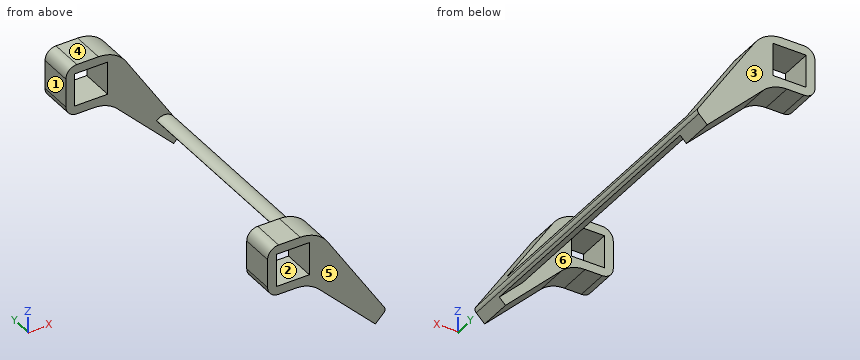
from build123d import *

# Parameters (mm, degrees)
SKETCH_1_W          = 15.000000000000002
SKETCH_1_H          = 15
EXTRUDE_1_DEPTH     = 160
CUT_EXTRUDE_2_DEPTH = 35
FILLET_3_R          = 5
FILLET_4_R          = 5
FILLET_6_R          = 15
FILLET_7_R          = 15
FILLET_8_R          = 15
FILLET_9_R          = 15
EXTRUDE_2_DEPTH     = 159
FILLET_10_R         = 5
FILLET_11_R         = 2


with BuildPart() as part:
    # Sketch 1 → Extrude 1 (new body)
    with BuildSketch(Plane(origin=(0, 0, 0), x_dir=(1, 0, 0), z_dir=(0, 1, 0))):
        Polygon((-11.5, 11.500000000000002), (7.5, 11.500000000000002), (37.49999999999999, 41.49999999999999), (42.44974746830583, 36.550252531694156), (11.5, -11.5), (-11.5, -11.5), align=None)
        Rectangle(SKETCH_1_W, SKETCH_1_H, mode=Mode.SUBTRACT)
    extrude(amount=EXTRUDE_1_DEPTH)

    # Sketch 4 → Cut-Extrude 2 (cut, symmetric)
    with BuildSketch(Plane(origin=(0, 0, -11.500000000000002), x_dir=(-1, 0, 0), z_dir=(0, 0, -1))):
        Polygon((-62.54884054332868, 145.00000000000003), (52.803582628705634, 145.00000000000003), (52.80358262870564, 15), (-62.548840543328666, 15), align=None)
    extrude(amount=CUT_EXTRUDE_2_DEPTH, both=True, mode=Mode.SUBTRACT)


with BuildPart() as cut_extrude_2_piece_1:
    # of the separate pieces the step leaves, piece 1, a body of its own (cut_extrude_2_pieces)
    add(part.part.solids().sort_by_distance((-11.5, 0, -11.5))[0])

    # Fillet 4
    fillet_4_edges = [cut_extrude_2_piece_1.edges().sort_by_distance(p)[0] for p in [
        (-11.5, 7.5, 11.5),
        (-11.5, 7.5, -11.500000000000002),
    ]]
    fillet(fillet_4_edges, radius=FILLET_4_R)

    # Fillet 7
    fillet_7_edges = [cut_extrude_2_piece_1.edges().sort_by_distance(p)[0] for p in [
        (11.5, 7.5, 11.5),
    ]]
    fillet(fillet_7_edges, radius=FILLET_7_R)

    # Fillet 8
    fillet_8_edges = [cut_extrude_2_piece_1.edges().sort_by_distance(p)[0] for p in [
        (7.5, 7.5, -11.500000000000002),
    ]]
    fillet(fillet_8_edges, radius=FILLET_8_R)



with BuildPart() as cut_extrude_2_piece_2:
    # of the separate pieces the step leaves, piece 2, a body of its own (cut_extrude_2_pieces)
    add(part.part.solids().sort_by_distance((7.5, 145, -11.5))[0])

    # Fillet 3
    fillet_3_edges = [cut_extrude_2_piece_2.edges().sort_by_distance(p)[0] for p in [
        (-11.5, 152.5, -11.500000000000002),
        (-11.5, 152.5, 11.5),
    ]]
    fillet(fillet_3_edges, radius=FILLET_3_R)

    # Fillet 6
    fillet_6_edges = [cut_extrude_2_piece_2.edges().sort_by_distance(p)[0] for p in [
        (11.5, 152.5, 11.5),
    ]]
    fillet(fillet_6_edges, radius=FILLET_6_R)

    # Fillet 9
    fillet_9_edges = [cut_extrude_2_piece_2.edges().sort_by_distance(p)[0] for p in [
        (7.5, 152.5, -11.500000000000002),
    ]]
    fillet(fillet_9_edges, radius=FILLET_9_R)


with BuildPart() as cut_extrude_2_piece_1_1:
    add(cut_extrude_2_piece_1.part)

    add(cut_extrude_2_piece_2.part)  # Extrude 2 merges Cut-Extrude 2 piece 2
    # Sketch 6 → Extrude 2 (add)
    with BuildSketch(Plane.XZ):
        Polygon((29.72182540693865, -28.064971157451247), (34.139072919876334, -23.647723644513547), (42.44974746830049, -36.550252531685864), (40.328427124736876, -38.671572875249474), align=None)
    extrude(amount=-EXTRUDE_2_DEPTH)

    # Fillet 10
    fillet_10_edges = [cut_extrude_2_piece_1_1.edges().sort_by_distance(p)[0] for p in [
        (34.139072919876334, 80.00000000000003, -23.647723644513547),
    ]]
    fillet(fillet_10_edges, radius=FILLET_10_R)

    # Fillet 11
    fillet_11_edges = [cut_extrude_2_piece_1_1.edges().sort_by_distance(p)[0] for p in [
        (42.449747468304494, 80, -36.55025253169208),
    ]]
    fillet(fillet_11_edges, radius=FILLET_11_R)


solid = cut_extrude_2_piece_1_1.part
The model under review builds one solid part; all positions refer to its coordinate system, in mm. Face numbers are marked on the shaded views. A direction names the side the tool comes from. Round coordinates to 2 decimals unless told otherwise and drop trailing zeros. Write each loop counter-clockwise with the first axis right and the second up, starting at its lowest first coordinate (ties: lowest second). Pieces come first, ordered by that corner, then holes. Notation, with made-up numbers: M -10,83.25 L 38,83.25 A25 ccw 38,103.25 Z; hole C -4,-39.75 d3. An arc over 180 degrees is marked long. Use a Markdown table: item, result. Add a question column.
Q1. To check wall thickness, follow line 1 (Y direction, x = 16.5, z = -14); line 2 (X direction, y = 12, z = -7); line 3 (X direction, y = 124.5, z = -34). State the ranges of each line that lie inside material, in increasing order.
Q2. We need section B-B, the plane z = -13. State the section outline as (x, y) points, plus the area to 3 significant figures.
Q3. Insertion check: pin 1 (6 mm diameter, centred on x = -1.5, y = 152, fed in from -Z); pin 2 (12 mm diameter, centred on x = -2.5, y = 4, fed in from -Z); pin 3 (16.5 mm diameter, centred on y = 11, z = 3, fed in from +X). Each pin has a flat end and moves straight along its axis. Give the tip position at first contact, or say it passes through.
Q4. We need section D-D, the plane z = -2. State the section outline as (x, y) points.
Q5. Machinability: for the marked faces 1 and 2, which of the approach directions +Z, -Z, +X, -X, +Y, -Y give a long, thin tool a straight path to every point of the face, cutting with its end or side? Answer none if there is none.
Q6. We need section A-A, the plane x = -0.5. State the section outline as (y, z) points.
Q7. The part is to be moulded in two halves that separate along Y. For the marked faces 3, 4, 5 and 6, say which applies: pulls with the +Y half, pulls with the -Y half, needs draft (parallel to the pull), parting line crosses it, or undercut.
Q8. We need section C-C, the plane y = 59.5. State the section outline as (x, z) points.
Findings below:
| question | item | result |
|---|---|---|
| 1 | line 1 | y = 0 to 15, 145 to 160 |
| 1 | line 2 | x = -11.47 to -7.5, 7.5 to 23.42 |
| 1 | line 3 | x = 35.66 to 40.81 |
| 2 | outline | M 7.83,0 L 27.28,0 L 27.28,15 L 7.83,15 Z; M 7.83,145 L 27.28,145 L 27.28,160 L 7.83,160 Z |
| 2 | area | 584 mm² |
| 3 | pin 1 | stops at z = -11.5 |
| 3 | pin 2 | stops at z = -11.66 |
| 3 | pin 3 | stops at x = 22.29 |
| 4 | outline | M -11.5,0 L -7.5,0 L -7.5,15 L -11.5,15 Z; M -11.5,145 L -7.5,145 L -7.5,160 L -11.5,160 Z; M 7.5,0 L 20.2,0 L 20.2,15 L 7.5,15 Z; M 7.5,145 L 20.2,145 L 20.2,160 L 7.5,160 Z |
| 5 | face 1 | +Z, -Z, -X, +Y, -Y |
| 5 | face 2 | +Y, -Y |
| 6 | outline | M 0,-11.5 L 15,-11.5 L 15,-7.5 L 0,-7.5 Z; M 0,7.5 L 15,7.5 L 15,11.5 L 0,11.5 Z; M 145,-11.5 L 160,-11.5 L 160,-7.5 L 145,-7.5 Z; M 145,7.5 L 160,7.5 L 160,11.5 L 145,11.5 Z |
| 7 | face 3 | pulls with the +Y half |
| 7 | face 4 | needs draft |
| 7 | face 5 | pulls with the -Y half |
| 7 | face 6 | undercut |
| 8 | outline | M 29.72,-28.06 L 40.33,-38.67 L 41.31,-37.69 A2 ccw 41.58,-35.19 L 37.5,-28.86 A5 ccw 29.76,-28.03 Z |
